Part model, mm, in its own coordinate system. Face numbers are marked on the shaded views. Coordinates: 2 decimals unless noted, no trailing zeros. Loops run counter-clockwise (first coordinate to the right, second up) from the corner with the lowest first, then second, coordinate; pieces in that order, holes last. Notation, with made-up numbers: (20.25, -12.75) - (39.25, -12.75) arc R31 ccw to (39.25, 25.25) - close; hole circle Ø10 at (20.25, 70.5). An arc over 180 degrees is marked (long way). Use a Markdown table: item, result. Add a question column.
1) Drop a flat-ended pin along its axis: P1, Ø6.5, axis at x = 12.5, y = -12.5, coming from the -Z side. Give the stop position or say it passes through.
2) Band-saw the part on B-B (y = -12.5). Give the cut face in (x, z), plus the area to 3 significant figures.
3) Probe probe 1 along Y at (x, z) = (12.5, 1); probe 2 along Y at (x, z) = (-9, 20); probe 3 along X at (y, z) = (15, 19). List the from-to ranges inside material, lowest first. Write a range as [from, to].
4) Band-saw the part on A-A (z = 18). Give the cut face in (x, y).
5) Pull direction Z, two halves, no side cores. Call the marked faces 1, 2 and 3: +Z half, -Z half, draft (parallel to the pull), parting line (faces both ways), or undercut.
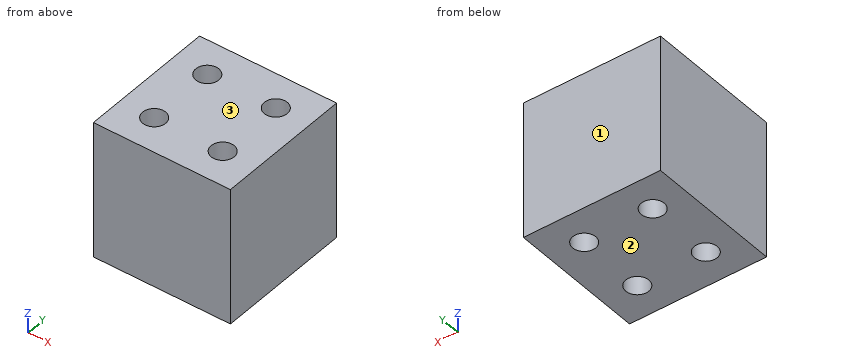
from build123d import *

# Parameters (mm, degrees)
F0_W     = 50
F0_H     = 50
F1_DEPTH = 25
F3_D     = 8.4


with BuildPart() as f1:
    # F0 (on Front) → F1 (new body, symmetric)
    with BuildSketch(Plane.XZ):
        Rectangle(F0_W, F0_H)
    extrude(amount=F1_DEPTH, both=True)

    # F3 (through all)
    with Locations(Plane.XY.offset(25)):
        with Locations((-12.5, 12.5), (12.5, 12.5), (12.5, -12.5), (-12.5, -12.5)):
            Hole(F3_D / 2)


solid = f1.part
Answer block:
| question | item | result |
|---|---|---|
| 1 | P1 | through |
| 2 | outline | (-25, -25) - (-16.7, -25) - (-16.7, 25) - (-25, 25) - close; (-8.3, -25) - (8.3, -25) - (8.3, 25) - (-8.3, 25) - close; (16.7, -25) - (25, -25) - (25, 25) - (16.7, 25) - close |
| 2 | area | 1,660 mm2 |
| 3 | probe 1 | [-25, -16.7], [-8.3, 8.3], [16.7, 25] |
| 3 | probe 2 | [-25, -14.82], [-10.18, 10.18], [14.82, 25] |
| 3 | probe 3 | [-25, -15.87], [-9.13, 9.13], [15.87, 25] |
| 4 | outline | (-25, -25) - (25, -25) - (25, 25) - (-25, 25) - close; hole circle Ø8.4 at (-12.5, -12.5); hole circle Ø8.4 at (-12.5, 12.5); hole circle Ø8.4 at (12.5, -12.5); hole circle Ø8.4 at (12.5, 12.5) |
| 5 | face 1 | draft |
| 5 | face 2 | -Z half |
| 5 | face 3 | +Z half |
